Part model, mm, in its own coordinate system. A direction names the side the tool comes from. Coordinates: 2 decimals unless noted, no trailing zeros. Loops run counter-clockwise (first coordinate to the right, second up) from the corner with the lowest first, then second, coordinate; pieces in that order, holes last. Notation, with made-up numbers: (75.25, 17.5) - (119.25, 17.5) arc R34 ccw to (119.25, 48.5) - close; hole circle Ø1 at (25, 11). An arc over 180 degrees is marked (long way). Use a Markdown table: item, result. Add a question column.
1) Pull direction Z, two halves, no side cores. Call faces 3 (the face through (2, 1244.6, -27)), 4 (the face through (13, 614, -48.26)), 5 (the face through (13, 614, -50.8)): +Z half, -Z half, draft (parallel to the pull), parting line (faces both ways), or undercut.
2) Band-saw the part on A-A (y = 924). Give the cut face in (x, z).
3) Probe probe 1 along Y at (x, z) = (12.7, -0.6) (3 decimals); probe 2 along X at (y, z) = (203, -32.5); probe 3 along Z at (x, y) = (1.35, 1212.85). List the from-to ranges inside material, lowest first. Write a range as [from, to].
4) Drop a flat-ended pin along its axis: P1, Ø7.5, axis at x = 17.46, y = 1095.92, coming from the +Z side. Give the stop position or say it passes through.
5) Tool access for faces 1 (the face through (22.86, 614, -25)), 2 (the face through (2, 0, -27)): list every direction of +Z, -Z, +X, -X, +Y, -Y with a clear straight run to the whole face (end or side of a thin tool).
from build123d import *

# Parameters (mm, degrees)
SKETCH1_W           = 25.4
SKETCH1_H           = 50.8
SKETCH1_W_2         = 20.32
SKETCH1_H_2         = 45.72
EXTRUDE_THIN1_DEPTH = 1244.6
SKETCH3_R           = 2.4892
SKETCH3_R_2         = 2.5019
CUT_EXTRUDE1_DEPTH  = 26.4
SKETCH4_R           = 2.4892
CUT_EXTRUDE2_DEPTH  = 26.4
SKETCH8_R           = 2.4892
CUT_EXTRUDE4_DEPTH  = 51.8
SKETCH11_R          = 2.4892
CUT_EXTRUDE6_DEPTH  = 51.8
SKETCH12_R          = 3.175
CUT_EXTRUDE7_DEPTH  = 51.8
SKETCH13_R          = 3.175
CUT_EXTRUDE8_DEPTH  = 51.8


with BuildPart() as part:
    # Sketch1 → Extrude-Thin1 (new body)
    with BuildSketch(Plane(origin=(0, 0, 0), x_dir=(1, 0, 0), z_dir=(0, 1, 0))):
        with Locations((12.7, 25.4)):
            Rectangle(SKETCH1_W, SKETCH1_H)
        with Locations((12.7, 25.4)):
            Rectangle(SKETCH1_W_2, SKETCH1_H_2, mode=Mode.SUBTRACT)
    extrude(amount=EXTRUDE_THIN1_DEPTH)

    # Sketch3 → Cut-Extrude1 (cut, through all)
    with BuildSketch(Plane(origin=(25.4, 0, 0), x_dir=(0, 0, -1), z_dir=(1, 0, 0))):
        with Locations((12.7, 12.7)):
            Circle(SKETCH3_R)
        with Locations((38.1, 12.960193373)):
            Circle(SKETCH3_R)
        with Locations((12.7, 721.632068306)):
            Circle(SKETCH3_R_2)
        with Locations((38.1, 721.632068306)):
            Circle(SKETCH3_R_2)
    extrude(amount=-CUT_EXTRUDE1_DEPTH, mode=Mode.SUBTRACT)

    # Sketch4 → Cut-Extrude2 (cut, through all)
    with BuildSketch(Plane.ZY):
        with Locations((-25.4, 1200.15)):
            Circle(SKETCH4_R)
        with Locations((-25.4, 1212.85)):
            Circle(SKETCH4_R)
    extrude(amount=-CUT_EXTRUDE2_DEPTH, mode=Mode.SUBTRACT)

    # Sketch8 → Cut-Extrude4 (cut, through all)
    with BuildSketch(Plane(origin=(0, 0, -50.8), x_dir=(-1, 0, 0), z_dir=(0, 0, -1))):
        with Locations((-12.7, 1084.8045868)):
            Circle(SKETCH8_R)
    extrude(amount=-CUT_EXTRUDE4_DEPTH, mode=Mode.SUBTRACT)

    # Sketch11 → Cut-Extrude6 (cut, through all)
    with BuildSketch(Plane.XY):
        with Locations((18.415, 12.7)):
            Circle(SKETCH11_R)
        with Locations((18.415, 25.4)):
            Circle(SKETCH11_R)
    extrude(amount=-CUT_EXTRUDE6_DEPTH, mode=Mode.SUBTRACT)

    # Sketch12 → Cut-Extrude7 (cut, through all)
    with BuildSketch(Plane(origin=(0, 0, -50.8), x_dir=(-1, 0, 0), z_dir=(0, 0, -1))):
        with Locations((-12.7, 1231.9)):
            Circle(SKETCH12_R)
    extrude(amount=-CUT_EXTRUDE7_DEPTH, mode=Mode.SUBTRACT)

    # Sketch13 → Cut-Extrude8 (cut, through all)
    with BuildSketch(Plane(origin=(0, 0, -50.8), x_dir=(-1, 0, 0), z_dir=(0, 0, -1))):
        with Locations((-17.4625, 1095.9170868)):
            Circle(SKETCH13_R)
        with Locations((-7.9375, 1073.6920868)):
            Circle(SKETCH13_R)
    extrude(amount=-CUT_EXTRUDE8_DEPTH, mode=Mode.SUBTRACT)


solid = part.part
Answer block:
| question | item | result |
|---|---|---|
| 1 | face 3 | draft |
| 1 | face 4 | undercut |
| 1 | face 5 | -Z half |
| 2 | outline | (0, -50.8) - (25.4, -50.8) - (25.4, 0) - (0, 0) - close; hole (2.54, -48.26) - (22.86, -48.26) - (22.86, -2.54) - (2.54, -2.54) - close |
| 3 | probe 1 | [0, 1082.315], [1087.294, 1228.725], [1235.075, 1244.6] |
| 3 | probe 2 | [0, 2.54], [22.86, 25.4] |
| 3 | probe 3 | [-50.8, -27.89], [-22.91, 0] |
| 4 | P1 | z = 0 |
| 5 | face 1 | +Y, -Y |
| 5 | face 2 | +Z, -Z, +X, -X, -Y |
